Verification items for this drawing (mm, ordinates from the low corner). Coordinates: 2 decimals unless noted, no trailing zeros. Loops run counter-clockwise (first coordinate to the right, second up) from the corner with the lowest first, then second, coordinate; pieces in that order, holes last.
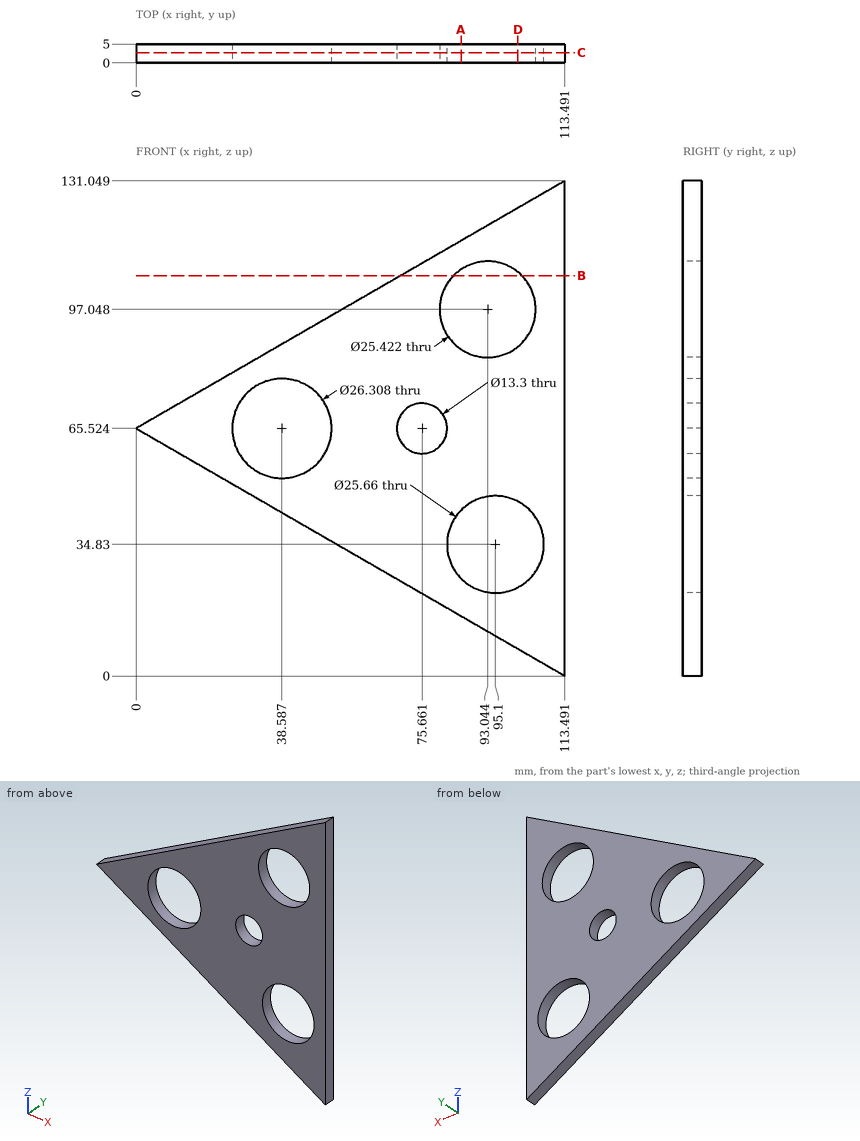
(1) Gauge pin test, flat ends, axial feed: P1, Ø12, axis at x = 75.66, z = 65.52, coming from the +Y side; P2, Ø1.5, axis at y = 3.5, z = 53.5, coming from the -X side (1 decimal); P3, Ø3, axis at x = 59.5, y = 1.5, coming from the +Z side. Record the tip position at first contact, or that the pin passes through.
(2) Section check B-B, the plane z = 106. Enter the section's corners in (x, y).
(3) Scan lines: line 1 along Z through (x, y) = (90, 4.3) (1 decimal); line 2 along Z through (x, y) = (85.5, 3) (1 decimal); line 3 along X through (y, z) = (0.25, 28.5) (1 decimal). Record each from-to range of solid material in increasing order.
(4) Section check A-A, the plane x = 86. Enter the section's corners in (y, z) (1 decimal), plus the area to 3 significant figures.
(5) Section check D-D, the plane x = 101. Enter the section's corners in (y, z) (1 decimal), plus the area to 3 significant figures.
(6) Section check C-C, the plane y = 2.75. Count the separate pieces of the cut face and the enclosed holes in it, plus the area to 3 significant figures.
Determined:
1. P1: passes through
1. P2: stops at x = 19.5
1. P3: stops at z = 100.74
2. outline: (70.11, 0) - (84.02, 0) - (84.02, 5) - (70.11, 5) - close; (102.07, 0) - (113.49, 0) - (113.49, 5) - (102.07, 5) - close
3. line 1: z = 13.6 to 23.1, 46.6 to 84.7, 109.4 to 117.5
3. line 2: z = 16.2 to 26.3, 43.3 to 86.8, 107.3 to 114.9
3. line 3: x = 64.1 to 83.9, 106.3 to 113.5
4. outline: (0, 15.9) - (5, 15.9) - (5, 25.8) - (0, 25.8) - close; (0, 43.9) - (5, 43.9) - (5, 86.5) - (0, 86.5) - close; (0, 107.6) - (5, 107.6) - (5, 115.2) - (0, 115.2) - close
4. area: 300 mm2
5. outline: (0, 7.2) - (5, 7.2) - (5, 23.4) - (0, 23.4) - close; (0, 46.2) - (5, 46.2) - (5, 87.1) - (0, 87.1) - close; (0, 107) - (5, 107) - (5, 123.8) - (0, 123.8) - close
5. area: 370 mm2
6. separate pieces: 1
6. enclosed holes: 4
6. area: 5,730 mm2
